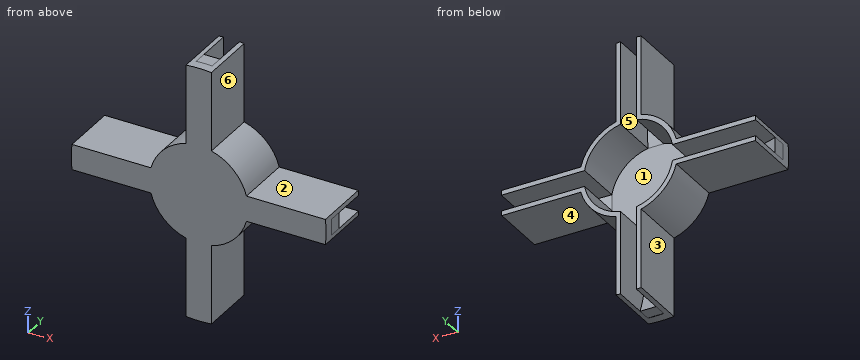
from build123d import *

# Parameters (mm, degrees)
SKETCH2_R           = 26.95
SKETCH2_R_2         = 9.45
BOSS_EXTRUDE2_DEPTH = 10
SKETCH3_R           = 26.95
BOSS_EXTRUDE3_DEPTH = 2
CUT_EXTRUDE1_DEPTH  = 10
BOSS_EXTRUDE4_DEPTH = 3.375
CIRPATTERN1_COUNT   = 4
CUT_EXTRUDE2_DEPTH  = 12
CIRPATTERN2_COUNT   = 4


with BuildPart() as part:
    # Sketch2 → Boss-Extrude2 (new body)
    with BuildSketch(Plane(origin=(0, 0, 0), x_dir=(1, 0, 0), z_dir=(0, 1, 0))):
        Circle(SKETCH2_R)
        Circle(SKETCH2_R_2, mode=Mode.SUBTRACT)
    extrude(amount=BOSS_EXTRUDE2_DEPTH)

    # Sketch3 → Boss-Extrude3 (add)
    with BuildSketch(Plane.XZ):
        Circle(SKETCH3_R)
    extrude(amount=BOSS_EXTRUDE3_DEPTH)

    # Sketch4 → Cut-Extrude1 (cut)
    with BuildSketch(Plane(origin=(0, 10, 0), x_dir=(1, 0, 0), z_dir=(0, 1, 0))):
        with BuildLine():
            Line((-1.6875, 26.8971159), (-1.6875, 9.298109687))
            ThreePointArc((-1.6875, 9.298109687), (0, 9.45), (1.6875, 9.298109687))
            Line((1.6875, 9.298109687), (1.6875, 26.8971159))
            ThreePointArc((1.6875, 26.8971159), (0, 26.95), (-1.6875, 26.8971159))
        make_face()
    cut_extrude1 = extrude(amount=-CUT_EXTRUDE1_DEPTH, mode=Mode.SUBTRACT)

    # Sketch7 → Boss-Extrude4 (add)
    with BuildSketch(Plane(origin=(-1.6875, 0, 0), x_dir=(0, 0, -1), z_dir=(1, 0, 0))):
        with BuildLine():
            Line((26.8971159, 0), (26.8971159, 2.834046352))
            add(Edge.make_bspline(
                [(9.298109687, 0), (19.523797501, 0), (26.8971159, 2.834046352)],
                knots=[4.71238898, 4.71238898, 4.71238898, 5.477856607, 5.477856607, 5.477856607], degree=2, weights=[1, 0.927647139, 1]))
            Line((9.298109687, 0), (26.8971159, 0))
        make_face()
    boss_extrude4 = extrude(amount=BOSS_EXTRUDE4_DEPTH)

    # CirPattern1: Cut-Extrude1, Boss-Extrude4 ×4 about axis
    cirpattern1_axis = Axis((0, 10, 0), (0, -1, 0))
    for i in range(1, CIRPATTERN1_COUNT):
        add(cut_extrude1.rotate(cirpattern1_axis, i * 360 / CIRPATTERN1_COUNT), mode=Mode.SUBTRACT)
        add(boss_extrude4.rotate(cirpattern1_axis, i * 360 / CIRPATTERN1_COUNT))

    # Sketch6 → Cut-Extrude2 (cut)
    with BuildSketch(Plane(origin=(0, 10, 0), x_dir=(1, 0, 0), z_dir=(0, 1, 0))):
        with BuildLine():
            Line((-26.815664149, 2.6875), (-10.098507006, 2.6875))
            ThreePointArc((-10.098507006, 2.6875), (-7.389265863, 7.389265863), (-2.6875, 10.098507006))
            Line((-2.6875, 10.098507006), (-2.6875, 26.815664149))
            ThreePointArc((-2.6875, 26.815664149), (-19.056527753, 19.056527753), (-26.815664149, 2.6875))
        make_face()
    cut_extrude2 = extrude(amount=-CUT_EXTRUDE2_DEPTH, mode=Mode.SUBTRACT)

    # CirPattern2: Cut-Extrude2 ×4 about axis
    cirpattern2_axis = Axis((0, 0, 0), (0, 1, 0))
    for i in range(1, CIRPATTERN2_COUNT):
        add(cut_extrude2.rotate(cirpattern2_axis, i * 360 / CIRPATTERN2_COUNT), mode=Mode.SUBTRACT)


solid = part.part
Verification items for the finished model (mm, model axes). Face numbers are marked on the shaded views. A direction names the side the tool comes from. Give positions to 0.01 mm unless a question says otherwise; leave off trailing zeros. Write each loop counter-clockwise with the first axis right and the second up, starting at its lowest first coordinate (ties: lowest second). Pieces come first, ordered by that corner, then holes. Notation, with made-up numbers: M -10,22 L 27,22 A9 ccw 27,37 Z; hole C 31.5,7 d9. An arc over 180 degrees is marked long. Use CSV: the item, a comma, the result in double quotes.
1) Cross-section at C-C (z = 3.5). Enter the section's corners in (x, y).
Final values:
outline,"M -9.85,-2 L 9.85,-2 L 9.85,10 L 8.78,10 L 8.78,0 L -8.78,0 L -8.78,10 L -9.85,10 Z"
2) Access from +Z, -Z, +X, -X, +Y, -Y to the whole of each face (thin tool, end or side, straight path). Record for the marked faces 4, 5 and 6.
Final values:
face 4,"-Z, +X, +Y, -Y"
face 5,"+Y"
face 6,"+Z, +X, +Y, -Y"
3) Cross-section at B-B (x = 6). Enter the section's corners in (y, z).
Final values:
outline,"M -2,-8.56 L 10,-8.56 L 10,-7.3 L 0,-7.3 L 0,7.3 L 10,7.3 L 10,8.56 L -2,8.56 Z"
4) Go/stop test with flat-tipped pins: pin 1 Ø9.5 at (x, z) = (1.5, -2.5) entering from +Y; pin 2 Ø3 at (y, z) = (2, -0.5) entering from +X; pin 3 Ø1.5 at (y, z) = (7.5, 8) entering from +X. Record where each tip stops, or that it passes through.
Final values:
pin 1,"y = 0"
pin 2,"x = 26.9"
pin 3,"x = 7.53"
5) Cross-section at A-A (y = 6). State how many separate pieces and enclosed holes the cut face has, plus the area to 3 significant figures.
Final values:
separate pieces,"4"
enclosed holes,"0"
area,"182 mm²"
6) Release check for a two-part mould opening along Z. For the marked faces 1, 2 and 3 record: released by +Z, released by -Z, zero draft, split by the parting line, or undercut.
Final values:
face 1,"undercut"
face 2,"released by +Z"
face 3,"zero draft"
7) Material ranges on line 1 along Z through (x, y) = (-12.5, 4.25); line 2 along X through (y, z) = (1, -22), recorded low to high.
Final values:
line 1,"-2.69 to -1.69, 1.69 to 2.69"
line 2,"-2.69 to 2.69"
